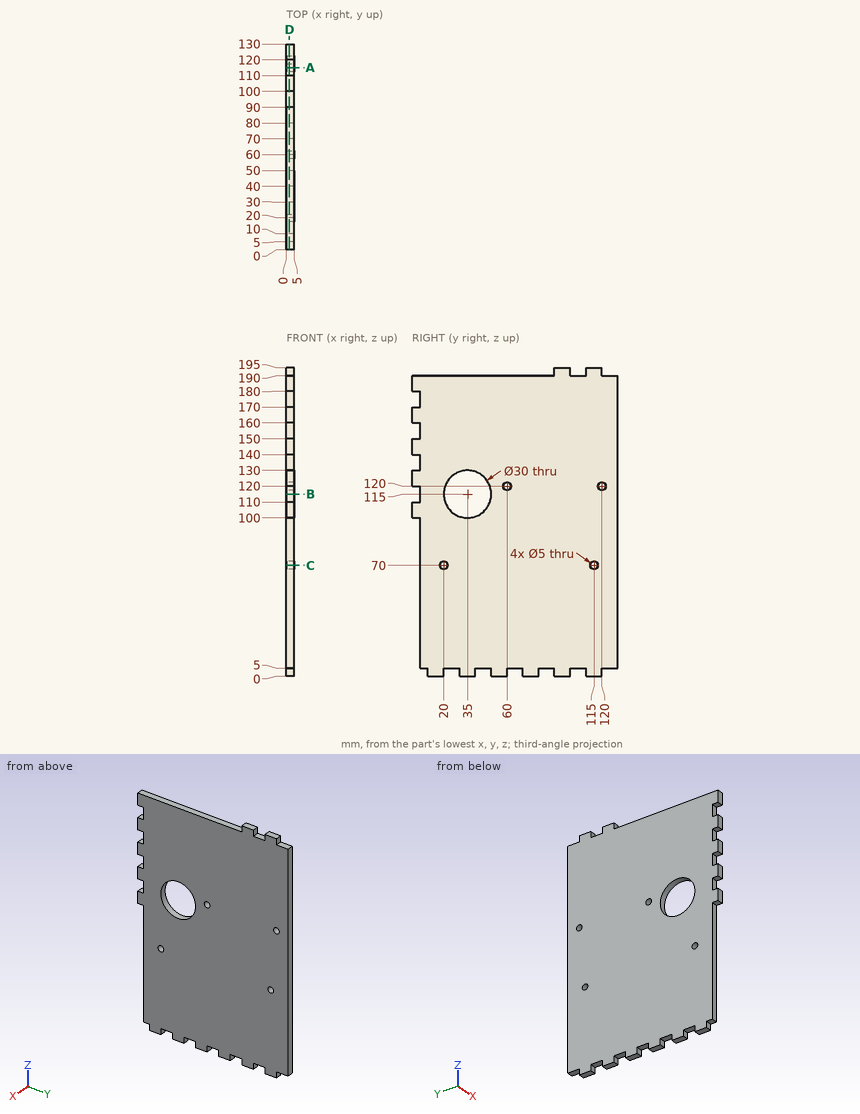
Can you work these out from the drawing? Everything is in mm from the part's minimum corner. Coordinates: 2 decimals unless noted, no trailing zeros. Write each loop counter-clockwise with the first axis right and the second up, starting at its lowest first coordinate (ties: lowest second). Pieces come first, ordered by that corner, then holes. Notation, with made-up numbers: (-39.5, -30) - (7.5, -30) arc R19 ccw to (7.5, 1) - close; hole circle Ø2 at (-21, 35). An arc over 180 degrees is marked (long way). Use a Markdown table: item, result.
Q1. Imagine slicing it at C-C (z = 70). List the corners of the cut face in (x, y) for me, and give its area (3 significant figures).
Geometry check:
| item | result |
|---|---|
| outline | (0, 5) - (5, 5) - (5, 17.5) - (0, 17.5) - close; (0, 22.5) - (5, 22.5) - (5, 112.5) - (0, 112.5) - close; (0, 117.5) - (5, 117.5) - (5, 130) - (0, 130) - close |
| area | 575 mm2 |
Q2. Imagine slicing it at D-D (x = 2.05). Count the separate pieces of the cut face and the enclosed holes in it, and give its area (3 significant figures).
Geometry check:
| item | result |
|---|---|
| separate pieces | 1 |
| enclosed holes | 5 |
| area | 23,000 mm2 |
Q3. Please list where these lines run through material, in increasing order: L1, parallel to Y at x = 2.4, z = 70; L2, parallel to Z at x = 2.95, y = 35; L3, parallel to Y at x = 3.1, z = 75.
Geometry check:
| item | result |
|---|---|
| L1 | y = 5 to 17.5, 22.5 to 112.5, 117.5 to 130 |
| L2 | z = 0 to 100, 130 to 190 |
| L3 | y = 5 to 130 |
Q4. Imagine slicing it at A-A (y = 115). List the corners of the cut face in (x, z) for me.
Geometry check:
| item | result |
|---|---|
| outline | (0, 0) - (5, 0) - (5, 67.5) - (0, 67.5) - close; (0, 72.5) - (5, 72.5) - (5, 195) - (0, 195) - close |
Q5. Imagine slicing it at B-B (z = 115). List the corners of the cut face in (x, y) for me, and give its area (3 significant figures).
Geometry check:
| item | result |
|---|---|
| outline | (0, 5) - (5, 5) - (5, 20) - (0, 20) - close; (0, 50) - (5, 50) - (5, 130) - (0, 130) - close |
| area | 475 mm2 |
Q6. I'm going to push flat-ended pins straight in: pin 1 Ø2.5 at (x, z) = (3, 3) entering from +Y; pin 2 Ø1 at (y, z) = (108, 127) entering from -X; pin 3 Ø1.5 at (x, y) = (2.5, 86.5) entering from -Z. Where does each tip first touch, or does it pass through?
Geometry check:
| item | result |
|---|---|
| pin 1 | stops at y = 120 |
| pin 2 | stops at x = 0 |
| pin 3 | stops at z = 5 |
